Autodesk Inventor part; units mm, degrees
ref_plane "YZ Plane" through (0, 0, 0) normal (1, 0, 0) x (0, 1, 0)
ref_plane "XZ Plane" through (0, 0, 0) normal (0, 1, 0) x (-1, 0, 0)
ref_plane "XY Plane" through (0, 0, 0) normal (0, 0, 1) x (1, 0, 0)
sketch "Sketch1" plane through (0, 0, 0) normal (0, 1, 0) x (-1, 0, 0)
  circle A0 centre (0, 0) radius 1.25
  line L0 (0, -3) -> (-2.5981, -1.5)
  line L1 (-2.5981, -1.5) -> (-2.5981, 1.5)
  line L2 (-2.5981, 1.5) -> (0, 3)
  line L3 (0, 3) -> (2.5981, 1.5)
  line L4 (2.5981, 1.5) -> (2.5981, -1.5)
  line L5 (2.5981, -1.5) -> (0, -3)
  dimension "d0" = 2.5
extrude "Extrusion1" add sketch "Sketch1" along normal blind 20
properties part number "Standoff-Hex-20mm"
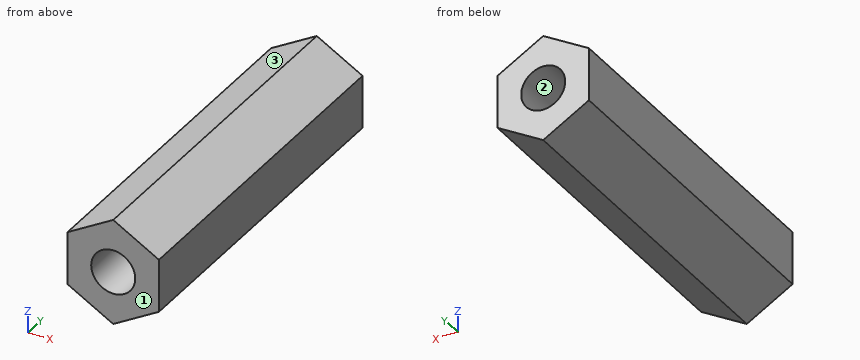
The listing builds one solid part. Answer for the finished solid, in the listing's coordinates (mm). Face numbers are marked on the shaded views. Round coordinates to 2 decimals unless told otherwise and drop trailing zeros. Loops run counter-clockwise (first coordinate to the right, second up) from the corner with the lowest first, then second, coordinate; pieces in that order, holes last. Notation, with made-up numbers: (50, 4.25) - (60, 4.25) arc R9 ccw to (60, 18.25) - close; hole circle Ø10 at (28.25, 62.25). An arc over 180 degrees is marked (long way). Return JSON: item names as keys, results as strings. Group by question number.
1. Consider probe 1 along X at (y, z) = (12.5, 0.05); probe 2 along X at (y, z) = (12.75, -0.65); probe 3 along Z at (x, y) = (0.3, 14.25). Determine where each line is inside the solid, lowest interval first.
2. The part is cut by section B-B on z = 0. Determine the outline of the cut face in (x, y), then the cut area to 3 significant figures.
3. The part is cut by section A-A on y = 15.75. Determine the outline of the cut face in (x, z), then the cut area to 3 significant figures.
4. Each of these flat-tipped pins is pushed along its axis until it touches: P1, Ø3, axis at x = 1.5, z = -2.5, coming from the -Y side; P2, Ø1.5, axis at x = -1, y = 11.5, coming from the +Z side. Where does it stop, or does it pass through?
5. The part is cut by section D-D on x = 1.85. Determine the outline of the cut face in (y, z), then the cut area to 3 significant figures.
6. The mould has two halves that part along Z. Classify the marked faces 1, 2 and 3: pulls with the +Z half, pulls with the -Z half, needs draft (parallel to the pull), parting line crosses it, or undercut.
7. The part is cut by section C-C on x = -0.95. Determine the outline of the cut face in (y, z), then the cut area to 3 significant figures.
Resolved:
{
 "1": {"probe 1": "x = -2.6 to -1.25, 1.25 to 2.6", "probe 2": "x = -2.6 to -1.07, 1.07 to 2.6", "probe 3": "z = -2.83 to -1.21, 1.21 to 2.83"},
 "2": {"outline": "(-2.6, 0) - (-1.25, 0) - (-1.25, 20) - (-2.6, 20) - close; (1.25, 0) - (2.6, 0) - (2.6, 20) - (1.25, 20) - close", "area": "53.9 mm²"},
 "3": {"outline": "(-2.6, -1.5) - (0, -3) - (2.6, -1.5) - (2.6, 1.5) - (0, 3) - (-2.6, 1.5) - close; hole circle Ø2.5 at (0, 0)", "area": "18.5 mm²"},
 "4": {"P1": "stops at y = 0", "P2": "stops at z = 2.86"},
 "5": {"outline": "(0, -1.93) - (20, -1.93) - (20, 1.93) - (0, 1.93) - close", "area": "77.3 mm²"},
 "6": {"face 1": "needs draft", "face 2": "undercut", "face 3": "pulls with the +Z half"},
 "7": {"outline": "(0, -2.45) - (20, -2.45) - (20, -0.81) - (0, -0.81) - close; (0, 0.81) - (20, 0.81) - (20, 2.45) - (0, 2.45) - close", "area": "65.6 mm²"}
}
